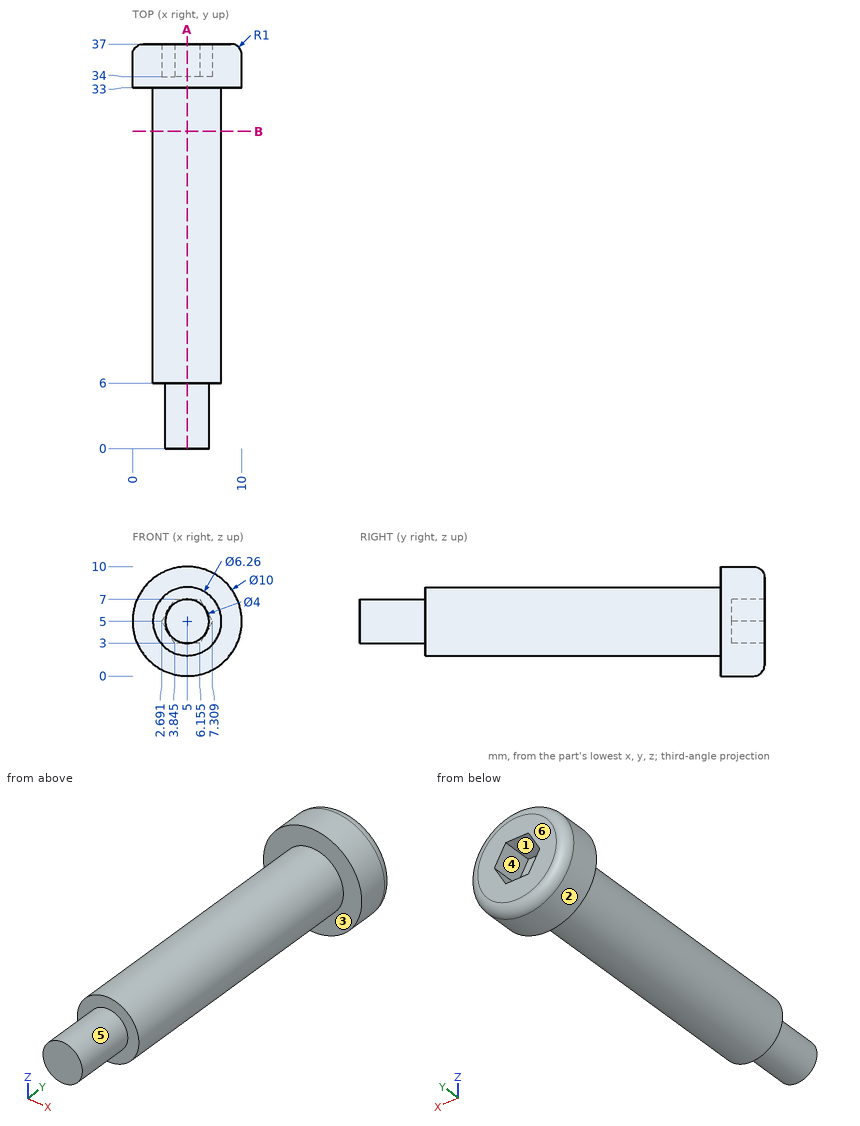
Study the drawing (mm; zero at the part's minimum x, y, z) and answer. A direction names the side the tool comes from. Round coordinates to 2 decimals unless told otherwise and drop trailing zeros. Loops run counter-clockwise (first coordinate to the right, second up) from the corner with the lowest first, then second, coordinate; pieces in that order, holes last. Notation, with made-up numbers: (27.5, 76.5) - (31.5, 76.5) arc R16 ccw to (31.5, 94.5) - close; hole circle Ø4 at (69, -16.75). An arc over 180 degrees is marked (long way). Use one line per item in the form item = value. Start each with the question number.
1. The part is cut by section B-B on y = 29. Determine the outline of the cut face in (x, z).
2. Given pin 1 Ø2 at (y, z) = (19, 7) entering from -X; pin 2 Ø3 at (x, z) = (8, 7) entering from -Y; pin 3 Ø4 at (y, z) = (31.5, 6.5) entering from -X, each flat-ended and moving along its own axis, determine where each tip first touches the part or whether it passes through.
3. A tool of negligible diameter and unlimited length cuts with its end or side. For the marked faces 1, 2 and 3, from which of +Z, -Z, +X, -X, +Y, -Y can it reach the whole face along a straight path? Write none if from no direction.
4. Consider line 1 (Y direction, x = 3.25, z = 2.5); line 2 (Y direction, x = 7, z = 1.5); line 3 (Z direction, x = 5.25, y = 10.5). Determine where each line is inside the solid, lowest interval first. Write a range as [from, to].
5. The part is cut by section A-A on x = 5. Determine the outline of the cut face in (y, z), then the cut area to 3 significant figures.
6. For a pull along Z with two mould halves and no side action, classify the marked faces 4, 5 and 6 as pulls with the +Z half, pulls with the -Z half, needs draft (parallel to the pull), parting line crosses it, or undercut.
Geometry check:
q1.outline = circle Ø6.26 at (5, 5)
q2.pin_1 = 2.03
q2.pin_2 = 6
q2.pin_3 = 0
q3.face_1 = +Y
q3.face_2 = +Y, -Y
q3.face_3 = -Y
q4.line_1 = [6, 37]
q4.line_2 = [33, 37]
q4.line_3 = [1.88, 8.12]
q5.outline = (0, 3) - (6, 3) - (6, 1.87) - (33, 1.87) - (33, 0) - (36, 0) arc R1 ccw to (37, 1) - (37, 3) - (34, 3) - (34, 7) - (37, 7) - (37, 9) arc R1 ccw to (36, 10) - (33, 10) - (33, 8.13) - (6, 8.13) - (6, 7) - (0, 7) - close
q5.area = 221 mm^2
q6.face_4 = undercut
q6.face_5 = parting line crosses it
q6.face_6 = needs draft
